The model under review builds one solid part; all positions refer to its coordinate system, in mm. A direction names the side the tool comes from. Coordinates: 2 decimals unless noted, no trailing zeros. Write each loop counter-clockwise with the first axis right and the second up, starting at its lowest first coordinate (ties: lowest second). Pieces come first, ordered by that corner, then holes. Notation, with made-up numbers: (44.25, 55.25) -> (102.25, 55.25) arc R22 ccw to (102.25, 63.25) -> close; hole circle Ø3 at (33, 15.25). An arc over 180 degrees is marked (long way). Write each question's results on one line, items separated by ' | '.
Autodesk Fusion 360 part; units mm, degrees
sketch "Sketch1" plane through (0, 0, 0) normal (0, 1, 0) x (1, 0, 0)
  line L0 (0, 0) -> (20, 0)
  line L1 (20, 0) -> (20, -20)
  line L2 (20, -20) -> (0, -20)
  line L3 (0, -20) -> (0, 0)
  dimension "d2" = 20
  dimension "d3" = 20
extrude "Extrude4" add sketch "Sketch1" along normal blind 20 makes body 1
extrude "Extrude1" add sketch "Sketch1" along normal blind 20 separate body makes body 2
sketch "Sketch2" plane through (0, 20, 0) normal (0, 1, 0) x (-1, 0, 0)
  line L0 (0, 20) -> (-20, 20)
  line L1 (-20, 20) -> (-20, 0)
  line L2 (-20, 0) -> (0, 0)
  line L3 (0, 0) -> (0, 20)
  line L4 (-20, 20) -> (0, 0) construction
  line L5 (0, 20) -> (-20, 0) construction
  circle A0 centre (-10, 10) radius 3.57
  circle A1 centre (-10, 10) radius 5.5
  dimension "d6" = 7.14
  dimension "d19" = 11
sketch "Sketch5" plane through (0, 0, 0) normal (-1, 0, 0) x (0, -1, 0)
  line L0 (0, 0) -> (0, 20)
  line L1 (0, 20) -> (-20, 20)
  line L2 (-20, 20) -> (-20, 0)
  line L3 (-20, 0) -> (0, 0)
sketch "Sketch6" plane through (20, 0, 0) normal (1, 0, 0) x (0, 1, 0)
  line L0 (0, 20) -> (0, 0)
  line L1 (0, 0) -> (20, 0)
  line L2 (20, 0) -> (20, 20)
  line L3 (20, 20) -> (0, 20)
  line L4 (0, 20) -> (20, 0) construction
  line L5 (20, 20) -> (0, 0) construction
  circle A0 centre (10, 10) radius 3.57
  circle A1 centre (10, 10) radius 5.5
  dimension "d14" = 7.14
  dimension "d20" = 11
extrude "Extrude5" cut sketch "Sketch6" against normal blind 20 contours A0 bodies 1 2
extrude "Extrude6" cut sketch "Sketch2" against normal blind 20 contours A0 bodies 1 2
extrude "Extrude7" cut sketch "Sketch2" against normal blind 16.97 contours A1 bodies 1 2
extrude "Extrude8" cut sketch "Sketch6" against normal blind 16.97 contours A1 bodies 1 2
sketch "Sketch8" plane through (0, 0, 20) normal (0, 0, 1) x (-1, 0, 0)
  line L0 (0, 0) -> (-20, 0)
  line L1 (-20, 0) -> (-20, -20)
  line L2 (-20, -20) -> (0, -20)
  line L3 (0, -20) -> (0, 0)
  line L4 (-20, 0) -> (-19, 0)
  line L5 (0, -20) -> (0, -19)
  line L6 (-20, 0) -> (-20, -1)
  line L7 (0, -20) -> (-1, -20)
  line L8 (-1, -20) -> (-20, -1)
  dimension "d27" = 1
  dimension "d28" = 1
  dimension "d29" = 1
  dimension "d30" = 1
extrude "Extrude9" cut sketch "Sketch8" against normal blind 21 contours L1 L2 L8 bodies 1 2
sketch "Sketch3" plane through (0, 0, 0) normal (1, 0, 0) x (0, 1, 0)
sketch "Sketch4" plane through (0, 0, 0) normal (-1, 0, 0) x (0, -1, 0)
  line L0 (0, 0) -> (0, 20)
  line L1 (0, 20) -> (-20, 20)
  line L2 (-20, 20) -> (-20, 0)
  line L3 (-20, 0) -> (0, 0)
  line L4 (0, 0) -> (-20, 20) construction
  line L5 (0, 20) -> (-20, 0) construction
  circle A0 centre (-10, 10) radius 3.57
  dimension "d7" = 7.14
extrude "Extrude2" [suppressed]
extrude "Extrude3" [suppressed]
hidden bodies 1
Q1. Add section D-D (x = 8). Write out the cut boundary in (y, z), plus the area to 3 significant figures.
Solution:
outline: (0, 0) -> (13, 0) -> (13, 4.88) -> (12, 4.88) arc R5.5 cw to (8, 4.88) -> (3.03, 4.88) -> (3.03, 7.04) -> (0, 7.04) -> close; (0, 12.96) -> (3.03, 12.96) -> (3.03, 15.12) -> (8, 15.12) arc R5.5 cw to (12, 15.12) -> (13, 15.12) -> (13, 20) -> (0, 20) -> close | area: 138 mm²
Q2. Add section B-B (x = 2.5). Write out the cut boundary in (y, z), plus the area to 3 significant figures.
Solution:
outline: (0, 0) -> (18.5, 0) -> (18.5, 20) -> (0, 20) -> close; hole circle Ø7.14 at (10, 10) | area: 330 mm²
Q3. Draft analysis for pull direction X (two halves, no side actions). For faces 4 (the flat face through (8, 8, 0)), 5 (the flat face through (0, 10, 6)), 6 (the flat face through (20, 0.5, 9.9)), 7 (the cylindrical face through (10.46, 1.54, 13.54)), state which applies: pulls with the +X half, pulls with the -X half, needs draft (parallel to the pull), parting line crosses it, or undercut.
Solution:
face 4: needs draft | face 5: pulls with the -X half | face 6: pulls with the +X half | face 7: undercut
Q4. Add section A-A (z = 10). Write out the cut boundary in (x, y).
Solution:
outline: (0, 0) -> (6.43, 0) -> (6.43, 3.03) -> (4.5, 3.03) -> (4.5, 4.5) -> (3.03, 4.5) -> (3.03, 6.43) -> (0, 6.43) -> close; (0, 13.57) -> (3.03, 13.57) -> (3.03, 15.5) -> (4.5, 15.5) -> (4.5, 16.5) -> (1, 20) -> (0, 20) -> close; (13.57, 0) -> (20, 0) -> (20, 1) -> (16.5, 4.5) -> (15.5, 4.5) -> (15.5, 3.03) -> (13.57, 3.03) -> close
Q5. Machinability: for faces 1 (the cylindrical face through (14.05, 5.01, 13.72)), 2 (the cylindrical face through (5.01, 5.95, 13.72)), 3 (the flat face through (10, 11, 17)), which of the approach directions +Z, -Z, +X, -X, +Y, -Y give a long, thin tool a straight path to every point of the face, cutting with its end or side? Answer none if there is none.
Solution:
face 1: +Y | face 2: +X | face 3: +Z, -Z, +X, +Y
Q6. Add section C-C (y = 9.5). Write out the cut boundary in (x, z).
Solution:
outline: (0, 0) -> (11.5, 0) -> (11.5, 4.52) -> (10.5, 4.52) arc R5.5 cw to (9.5, 4.52) -> (3.03, 4.52) -> (3.03, 6.47) -> (0, 6.47) -> close; (0, 13.53) -> (3.03, 13.53) -> (3.03, 15.48) -> (9.5, 15.48) arc R5.5 cw to (10.5, 15.48) -> (11.5, 15.48) -> (11.5, 20) -> (0, 20) -> close
Q7. Clearance check with flat-ended pins moving along their axes: P1, Ø3.5, axis at x = 8.5, z = 12, coming from the +Y side; P2, Ø9, axis at y = 10, z = 10, coming from the -X side; P3, Ø9, axis at y = 8.5, z = 9.5, coming from the +X side; P4, Ø11.5, axis at x = 10, z = 10, coming from the +Y side. State where each tip first meets the part, or that it passes through.
Solution:
P1: y = 3.03 | P2: x = 0 | P3: x = 17 | P4: y = 16.75
Q8. For line 1 (Z direction, x = 1.65, y = 10); line 2 (X direction, y = 10.75, z = 15); line 3 (Z direction, x = 5.75, y = 10), list the stretches that pass through material, from the lowest coordinate up. Write a range as from..to.
Solution:
line 1: 0..6.43, 13.57..20 | line 2: 0..3.03 | line 3: 0..4.5, 15.5..20
